Check sheet for the modelled part. Datum: model origin and axes. Units: mm. A direction names the side the tool comes from. Round coordinates to 2 decimals unless told otherwise and drop trailing zeros. Order: outer loops, then holes, each group sorted by start corner. A loop starts at its lowest first (then second) coordinate and runs counter-clockwise, first axis right, second up. Notation, with made-up numbers: (2, 31) -> (55, 31) arc R11 cw to (55, 45) -> close; hole circle Ø6 at (17.5, 36). An arc over 180 degrees is marked (long way). Answer in a Markdown table with one row per item.
from build123d import *
from build123d import SkipClean  # not in build123d's __all__

# Parameters (mm, degrees)
F0_R     = 63.5754098613
F1_DEPTH = 25
F2_R     = 10
F3_DEPTH = 25.001
F4_W     = 50
F4_H     = 50
F4_R     = 10
F5_DEPTH = 25
F6_W     = 7.0136869326
F6_H     = 12.901866436
F7_DEPTH = 25
F8_COUNT = 10


# Not quite as in the source:
# - after a boolean that leaves OpenCascade's solid faulty, fix() repairs it


with BuildPart() as f1:
    # F0 (on Front) → F1 (new body)
    with BuildSketch(Plane.XZ):
        Circle(F0_R)
    extrude(amount=F1_DEPTH)

    # F2 (on face) → F3 (cut, through all)
    with BuildSketch(Plane(origin=(0, 0, 0), x_dir=(-1, 0, 0), z_dir=(0, 1, 0))):
        Circle(F2_R)
    extrude(amount=-F3_DEPTH, mode=Mode.SUBTRACT)

    # F4 (on face) → F5 (join)
    with BuildSketch(Plane.XZ.offset(25)):
        Rectangle(F4_W, F4_H)
        Circle(F4_R, mode=Mode.SUBTRACT)
    with SkipClean():  # cleaning this boolean's faces spoils the solid; the shape is the same uncleaned
        extrude(amount=F5_DEPTH)

    # F6 (on face) → F7 (join)
    with BuildSketch(Plane(origin=(0, 0, 0), x_dir=(-1, 0, 0), z_dir=(0, 1, 0))):
        with Locations((0, -50)):
            Rectangle(F6_W, F6_H)
    f7 = extrude(amount=F7_DEPTH)

    add(f1.part.fix(), mode=Mode.REPLACE)

    # F8: F7 ×10 about axis
    f8_axis = Axis((0, 0, 0), (0, -1, 0))
    for i in range(1, F8_COUNT):
        add(f7.rotate(f8_axis, i * 360 / F8_COUNT), clean=False)


solid = f1.part
Item 1: Cross-section at B-B (y = -34.5). Record the boundary of the cut face in (x, z), and give its area (3 significant figures).
Result sheet:
| item | result |
|---|---|
| outline | (-25, -25) -> (25, -25) -> (25, 25) -> (-25, 25) -> close; hole circle Ø20 at (0, 0) |
| area | 2,190 mm^2 |
Item 2: Scan lines: line 1 (X direction, y = -38.75, z = 0); line 2 (Y direction, x = 19, z = 43). Record each from-to range of solid material in increasing order. Write a range as [from, to].
Result sheet:
| item | result |
|---|---|
| line 1 | x = [-25, -10], [10, 25] |
| line 2 | y = [-25, 0] |
Item 3: Mould release check, pull along Z, two halves, no side actions. Record for faces 1 (the flat face through (32.279, 12.325, 38.463)), 2 (the flat face through (-48.722, 12.325, 12.144)), 3 (the flat face through (29, 25, -40)), 4 (the flat face through (33.22, 12.32, -45.64)): pulls with the +Z half, pulls with the -Z half, needs draft (parallel to the pull), parting line crosses it, or undercut.
Result sheet:
| item | result |
|---|---|
| face 1 | undercut |
| face 2 | undercut |
| face 3 | needs draft |
| face 4 | pulls with the -Z half |
Item 4: Depth check by flat-ended pin: P1, Ø4, axis at y = 15, z = 50, coming from the +X side; P2, Ø2, axis at x = 1.5, y = 8.5, coming from the +Z side; P3, Ø5, axis at x = 42.5, y = 16, coming from the +Z side; P4, Ø12, axis at x = 0, z = 0, coming from the -Y side. Enter the tip coordinate at first touch or a pass-through.
Result sheet:
| item | result |
|---|---|
| P1 | stops at x = 3.51 |
| P2 | stops at z = 56.45 |
| P3 | stops at z = 18.31 |
| P4 | passes through |
Item 5: Cross-section at A-A (x = 0). Record the boundary of the cut face in (y, z), and give its area (3 significant figures).
Result sheet:
| item | result |
|---|---|
| outline | (-50, -25) -> (-25, -25) -> (-25, -63.58) -> (0, -63.58) -> (0, -56.45) -> (25, -56.45) -> (25, -43.55) -> (0, -43.55) -> (0, -10) -> (-50, -10) -> close; (-50, 10) -> (0, 10) -> (0, 43.55) -> (25, 43.55) -> (25, 56.45) -> (0, 56.45) -> (0, 63.58) -> (-25, 63.58) -> (-25, 25) -> (-50, 25) -> close |
| area | 4,070 mm^2 |
Item 6: Cross-section at C-C (z = 0). Record the boundary of the cut face in (x, y).
Result sheet:
| item | result |
|---|---|
| outline | (-63.58, -25) -> (-25, -25) -> (-25, -50) -> (-10, -50) -> (-10, 0) -> (-63.58, 0) -> close; (10, -50) -> (25, -50) -> (25, -25) -> (63.58, -25) -> (63.58, 0) -> (10, 0) -> close |
Item 7: Set-up check for faces 5 (the flat face through (48.722, 12.325, -12.144)), 6 (the flat face through (53.673, 12.325, 17.491)), 7 (the flat face through (-33.14, 12.32, -45.7)): record each of +Z, -Z, +X, -X, +Y, -Y from which the full face is reachable in a straight line by a thin tool's end or side.
Result sheet:
| item | result |
|---|---|
| face 5 | +X, +Y |
| face 6 | +Z, +X, +Y |
| face 7 | -Z, -X, +Y |
Item 8: Cross-section at D-D (y = 9). State how many separate pieces and enclosed holes the cut face has, and give its area (3 significant figures).
Result sheet:
| item | result |
|---|---|
| separate pieces | 10 |
| enclosed holes | 0 |
| area | 905 mm^2 |
